Check sheet for the modelled part. Datum: model origin and axes. Units: mm. A direction names the side the tool comes from. Give positions to 0.01 mm unless a question says otherwise; leave off trailing zeros. Order: outer loops, then holes, each group sorted by start corner. A loop starts at its lowest first (then second) coordinate and runs counter-clockwise, first axis right, second up. Notation, with made-up numbers: (87, 57.5) -> (139, 57.5) arc R25 cw to (139, 79.5) -> close; hole circle Ø4 at (24.25, 28.5). An arc over 180 degrees is marked (long way). One line per question, with ' | ' between items.
```python
from build123d import *

# Parameters (mm, degrees)
SKETCH1_R           = 12.5
SKETCH1_R_2         = 1
SKETCH1_R_3         = 1.5
SKETCH1_R_4         = 1.6
BOSS_EXTRUDE1_DEPTH = 5
SKETCH2_R           = 2
CUT_EXTRUDE1_DEPTH  = 2


with BuildPart() as part:
    # Sketch1 → Boss-Extrude1 (new body)
    with BuildSketch(Plane(origin=(0, 0, 0), x_dir=(1, 0, 0), z_dir=(0, 1, 0))):
        with Locations(Location((0, 0, 0), (0, 0, 270))):
            Circle(SKETCH1_R)
        with Locations(Location((0, -8, 0), (0, 0, 270))):
            Circle(SKETCH1_R_2, mode=Mode.SUBTRACT)
        with Locations(Location((0, 8, 0), (0, 0, 270))):
            Circle(SKETCH1_R_2, mode=Mode.SUBTRACT)
        with Locations(Location((0, 0, 0), (0, 0, 270))):
            Circle(SKETCH1_R_3, mode=Mode.SUBTRACT)
        with Locations(Location((-10.5, 0, 0), (0, 0, 270))):
            Circle(SKETCH1_R_4, mode=Mode.SUBTRACT)
        with Locations(Location((7.5, 0, 0), (0, 0, 270))):
            Circle(SKETCH1_R_4, mode=Mode.SUBTRACT)
    extrude(amount=BOSS_EXTRUDE1_DEPTH)

    # Sketch2 → Cut-Extrude1 (cut)
    with BuildSketch(Plane(origin=(0, 5, 0), x_dir=(1, 0, 0), z_dir=(0, 1, 0))):
        with Locations(Location((0, 8, 0), (0, 0, 270))):
            Circle(SKETCH2_R)
        with Locations(Location((0, -8, 0), (0, 0, 270))):
            Circle(SKETCH2_R)
    extrude(amount=-CUT_EXTRUDE1_DEPTH, mode=Mode.SUBTRACT)


solid = part.part
```
Q1. Access from +Z, -Z, +X, -X, +Y, -Y to the whole of each face (thin tool, end or side, straight path). Record for faces 1 (the face through (-1, 3, 9)), 2 (the face through (5.94, 2.46, -0.35)).
Result sheet:
face 1: +Y | face 2: +Y, -Y
Q2. Mould release check, pull along X, two halves, no side actions. Record for faces 3 (the face through (0, 5, 3)), 4 (the face through (3.755, 2.465, 11.923)), 5 (the face through (-0.6, 1.5, -8.8)), 6 (the face through (0.45, 2.46, 1.43)): pulls with the +X half, pulls with the -X half, needs draft (parallel to the pull), parting line crosses it, or undercut.
Result sheet:
face 3: needs draft | face 4: parting line crosses it | face 5: undercut | face 6: undercut
Q3. Section check A-A (y = 1.15). Enter the section's corners in (x, z), and give its area (3 significant figures).
Result sheet:
outline: circle Ø25 at (0, 0); hole circle Ø3.2 at (-10.5, 0); hole circle Ø3 at (0, 0); hole circle Ø2 at (0, -8); hole circle Ø2 at (0, 8); hole circle Ø3.2 at (7.5, 0) | area: 461 mm2
Q4. Section check C-C (x = 8.75). Enter the section's corners in (y, z), and give its area (3 significant figures).
Result sheet:
outline: (0, -8.93) -> (5, -8.93) -> (5, -1) -> (0, -1) -> close; (0, 1) -> (5, 1) -> (5, 8.93) -> (0, 8.93) -> close | area: 79.3 mm2
Q5. Section check B-B (z = 8). Enter the section's corners in (x, y).
Result sheet:
outline: (-9.6, 0) -> (-1, 0) -> (-1, 3) -> (-2, 3) -> (-2, 5) -> (-9.6, 5) -> close; (1, 0) -> (9.6, 0) -> (9.6, 5) -> (2, 5) -> (2, 3) -> (1, 3) -> close
Q6. Depth check by flat-ended pin: pin 1 Ø1.5 at (x, y) = (2.5, 1) entering from +Z; pin 2 Ø1.2 at (x, z) = (-0.5, -7.5) entering from +Y. Enter the tip coordinate at first touch or a pass-through.
Result sheet:
pin 1: stops at z = 12.38 | pin 2: stops at y = 3
Q7. Thickness scan on line 1 (Z direction, x = -0.5, y = 1); line 2 (Z direction, x = -0.75, y = 1.25); line 3 (X direction, y = 0.55, z = -0.5). Record the ranges inside material, lowest first.
Result sheet:
line 1: z = -12.49 to -8.87, -7.13 to -1.41, 1.41 to 7.13, 8.87 to 12.49 | line 2: z = -12.48 to -8.66, -7.34 to -1.3, 1.3 to 7.34, 8.66 to 12.48 | line 3: x = -12.49 to -12.02, -8.98 to -1.41, 1.41 to 5.98, 9.02 to 12.49
Q8. Section check D-D (z = -0.25). Enter the section's corners in (x, y), and give its area (3 significant figures).
Result sheet:
outline: (-12.5, 0) -> (-12.08, 0) -> (-12.08, 5) -> (-12.5, 5) -> close; (-8.92, 0) -> (-1.48, 0) -> (-1.48, 5) -> (-8.92, 5) -> close; (1.48, 0) -> (5.92, 0) -> (5.92, 5) -> (1.48, 5) -> close; (9.08, 0) -> (12.5, 0) -> (12.5, 5) -> (9.08, 5) -> close | area: 78.6 mm2
